Verification items for the finished model (mm, model axes). Round coordinates to 2 decimals unless told otherwise and drop trailing zeros. Loops run counter-clockwise (first coordinate to the right, second up) from the corner with the lowest first, then second, coordinate; pieces in that order, holes last. Notation, with made-up numbers: M -15,86 L 3,86 A18 cw 3,98 Z; hole C -39,35.25 d10. An arc over 180 degrees is marked long. Answer as CSV lines item,"result".
```python
from build123d import *
from OCP.BRepFilletAPI import BRepFilletAPI_MakeChamfer

# Parameters (mm, degrees)
BOSS_EXTRUDE1_DEPTH = 2.4
SKETCH2_R           = 2
CUT_EXTRUDE1_DEPTH  = 31.907209919
CHAMFER1_SIZE       = 2.38
CHAMFER1_SIZE2      = 1.109812226
SKETCH3_R           = 12.7
SKETCH3_R_2         = 11.375
BOSS_EXTRUDE2_DEPTH = 18
CUT_EXTRUDE2_START  = -30
SKETCH4_R           = 11.375
CUT_EXTRUDE2_DEPTH  = 30
CHAMFER2_SIZE       = 2.4293521
CHAMFER2_SIZE_2     = 3
CHAMFER3_SIZE       = 1.619568066
CHAMFER3_SIZE_2     = 2
CUT_EXTRUDE3_DEPTH  = 37.954778273


with BuildPart() as part:
    # Sketch1 → Boss-Extrude1 (new body)
    with BuildSketch(Plane.XY):
        with BuildLine():
            Line((6.35, 28.075), (-6.35, 28.075))
            ThreePointArc((-6.35, 28.075), (-10.840128061, 26.215128061), (-12.7, 21.725))
            Line((-12.7, 21.725), (-12.7, -21.725))
            ThreePointArc((-12.7, -21.725), (-10.840128061, -26.215128061), (-6.35, -28.075))
            Line((-6.35, -28.075), (6.35, -28.075))
            ThreePointArc((6.35, -28.075), (10.840128061, -26.215128061), (12.7, -21.725))
            Line((12.7, -21.725), (12.7, 21.725))
            ThreePointArc((12.7, 21.725), (10.840128061, 26.215128061), (6.35, 28.075))
        make_face()
    extrude(amount=BOSS_EXTRUDE1_DEPTH)

    # Sketch2 → Cut-Extrude1 (cut, through all)
    with BuildSketch(Plane(origin=(0, 0, 0), x_dir=(-1, 0, 0), z_dir=(0, 0, -1))):
        with Locations((-7.7, 20.1248)):
            Circle(SKETCH2_R)
        with Locations((-7.7, -20.125)):
            Circle(SKETCH2_R)
        with Locations((7.7, 20.125)):
            Circle(SKETCH2_R)
        with Locations((7.7, -20.125)):
            Circle(SKETCH2_R)
    extrude(amount=-CUT_EXTRUDE1_DEPTH, mode=Mode.SUBTRACT)

    # Chamfer1: one chamfer whose edges measure the first distance from different faces: ONE call of the kernel's chamfer builder (chamfer() names one face for all edges)
    chamfer1_edges_1 = [part.edges().sort_by_distance(p)[0] for p in [
        (-10.840128061, 26.215128061, 2.4),
    ]]
    chamfer1_side_1 = [part.faces().sort_by_distance(p)[0] for p in [
        (-10.840128061, 26.215128061, 1.2),
    ]]
    chamfer1_edges_2 = [part.edges().sort_by_distance(p)[0] for p in [
        (-12.7, 0, 2.4),
    ]]
    chamfer1_side_2 = [part.faces().sort_by_distance(p)[0] for p in [
        (-12.7, 0, 1.2),
    ]]
    chamfer1_edges_3 = [part.edges().sort_by_distance(p)[0] for p in [
        (-10.840128061, -26.215128061, 2.4),
    ]]
    chamfer1_side_3 = [part.faces().sort_by_distance(p)[0] for p in [
        (-10.840128061, -26.215128061, 1.2),
    ]]
    chamfer1_edges_4 = [part.edges().sort_by_distance(p)[0] for p in [
        (0, -28.075, 2.4),
    ]]
    chamfer1_side_4 = [part.faces().sort_by_distance(p)[0] for p in [
        (0, -28.075, 1.2),
    ]]
    chamfer1_edges_5 = [part.edges().sort_by_distance(p)[0] for p in [
        (10.840128061, -26.215128061, 2.4),
    ]]
    chamfer1_side_5 = [part.faces().sort_by_distance(p)[0] for p in [
        (10.840128061, -26.215128061, 1.2),
    ]]
    chamfer1_edges_6 = [part.edges().sort_by_distance(p)[0] for p in [
        (12.7, 0, 2.4),
    ]]
    chamfer1_side_6 = [part.faces().sort_by_distance(p)[0] for p in [
        (12.7, 0, 1.2),
    ]]
    chamfer1_edges_7 = [part.edges().sort_by_distance(p)[0] for p in [
        (10.840128061, 26.215128061, 2.4),
    ]]
    chamfer1_side_7 = [part.faces().sort_by_distance(p)[0] for p in [
        (10.840128061, 26.215128061, 1.2),
    ]]
    chamfer1_edges_8 = [part.edges().sort_by_distance(p)[0] for p in [
        (0, 28.075, 2.4),
    ]]
    chamfer1_side_8 = [part.faces().sort_by_distance(p)[0] for p in [
        (0, 28.075, 1.2),
    ]]
    chamfer1 = BRepFilletAPI_MakeChamfer(part.part.solid().wrapped)
    for e in chamfer1_edges_1:
        chamfer1.Add(CHAMFER1_SIZE, CHAMFER1_SIZE2, e.wrapped, chamfer1_side_1[0].wrapped)  # the first distance lies on this face
    for e in chamfer1_edges_2:
        chamfer1.Add(CHAMFER1_SIZE, CHAMFER1_SIZE2, e.wrapped, chamfer1_side_2[0].wrapped)  # the first distance lies on this face
    for e in chamfer1_edges_3:
        chamfer1.Add(CHAMFER1_SIZE, CHAMFER1_SIZE2, e.wrapped, chamfer1_side_3[0].wrapped)  # the first distance lies on this face
    for e in chamfer1_edges_4:
        chamfer1.Add(CHAMFER1_SIZE, CHAMFER1_SIZE2, e.wrapped, chamfer1_side_4[0].wrapped)  # the first distance lies on this face
    for e in chamfer1_edges_5:
        chamfer1.Add(CHAMFER1_SIZE, CHAMFER1_SIZE2, e.wrapped, chamfer1_side_5[0].wrapped)  # the first distance lies on this face
    for e in chamfer1_edges_6:
        chamfer1.Add(CHAMFER1_SIZE, CHAMFER1_SIZE2, e.wrapped, chamfer1_side_6[0].wrapped)  # the first distance lies on this face
    for e in chamfer1_edges_7:
        chamfer1.Add(CHAMFER1_SIZE, CHAMFER1_SIZE2, e.wrapped, chamfer1_side_7[0].wrapped)  # the first distance lies on this face
    for e in chamfer1_edges_8:
        chamfer1.Add(CHAMFER1_SIZE, CHAMFER1_SIZE2, e.wrapped, chamfer1_side_8[0].wrapped)  # the first distance lies on this face
    add(Compound.cast(chamfer1.Shape()), mode=Mode.REPLACE)

    # Sketch3 → Boss-Extrude2 (add)
    with BuildSketch(Plane(origin=(0, 0, 0), x_dir=(-1, 0, 0), z_dir=(0, 0, -1))):
        Circle(SKETCH3_R)
        Circle(SKETCH3_R_2, mode=Mode.SUBTRACT)
    extrude(amount=BOSS_EXTRUDE2_DEPTH)

    # Sketch4 → Cut-Extrude2 (cut)
    with BuildSketch(Plane(origin=(0, 0, 0), x_dir=(-1, 0, 0), z_dir=(0, 0, -1)).offset(CUT_EXTRUDE2_START)):
        Circle(SKETCH4_R)
    extrude(amount=CUT_EXTRUDE2_DEPTH, mode=Mode.SUBTRACT)

    # Chamfer2
    # the kernel refuses this chamfer: 3, 2.4293521 mm, written as the material it takes off along each edge
    with BuildSketch(Plane(origin=(7.7, -20.125, 2.4), x_dir=(-1, 0, 0), z_dir=(0, -1, 0))) as chamfer2_piece_1:
        Polygon((2 + CHAMFER2_SIZE, 0), (2, CHAMFER2_SIZE_2), (2, 0), align=None)
    revolve(axis=Axis((7.7, -20.125, 2.4), (0, 0, -1)), mode=Mode.SUBTRACT)
    with BuildSketch(Plane(origin=(-7.7, -20.125, 2.4), x_dir=(-1, 0, 0), z_dir=(0, -1, 0))) as chamfer2_piece_2:
        Polygon((2 + CHAMFER2_SIZE, 0), (2, CHAMFER2_SIZE_2), (2, 0), align=None)
    revolve(axis=Axis((-7.7, -20.125, 2.4), (0, 0, -1)), mode=Mode.SUBTRACT)
    with BuildSketch(Plane(origin=(7.7, 20.1248, 2.4), x_dir=(-1, 0, 0), z_dir=(0, -1, 0))) as chamfer2_piece_3:
        Polygon((2 + CHAMFER2_SIZE, 0), (2, CHAMFER2_SIZE_2), (2, 0), align=None)
    revolve(axis=Axis((7.7, 20.1248, 2.4), (0, 0, -1)), mode=Mode.SUBTRACT)
    with BuildSketch(Plane(origin=(-7.7, 20.125, 2.4), x_dir=(-1, 0, 0), z_dir=(0, -1, 0))) as chamfer2_piece_4:
        Polygon((2 + CHAMFER2_SIZE, 0), (2, CHAMFER2_SIZE_2), (2, 0), align=None)
    revolve(axis=Axis((-7.7, 20.125, 2.4), (0, 0, -1)), mode=Mode.SUBTRACT)

    # Chamfer3
    # the kernel refuses this chamfer: 2, 1.619568066 mm, written as the material it takes off along each edge
    with BuildSketch(Plane(origin=(0, 0, 2.4), x_dir=(-1, 0, 0), z_dir=(0, 1, 0))) as chamfer3_piece_1:
        Polygon((11.375 + CHAMFER3_SIZE, 0), (11.375, -CHAMFER3_SIZE_2), (11.375, 0), align=None)
    revolve(axis=Axis((0, 0, 2.4), (0, 0, 1)), mode=Mode.SUBTRACT)

    # Sketch5 → Cut-Extrude3 (cut, through all)
    with BuildSketch(Plane(origin=(0, 0, -18), x_dir=(-1, 0, 0), z_dir=(0, 0, -1))):
        with BuildLine():
            Line((-0.85, 11.343197301), (-0.85, 12.75))
            Line((-0.85, 12.75), (0.85, 12.75))
            Line((0.85, 12.75), (0.85, 11.343197301))
            ThreePointArc((0.85, 11.343197301), (0, 11.375), (-0.85, 11.343197301))
        make_face()
    extrude(amount=-CUT_EXTRUDE3_DEPTH, mode=Mode.SUBTRACT)


solid = part.part
```
1) Section check A-A (x = 0). Record the cut outline in (y, z) (3 decimals), plus the area to 3 significant figures.
Here are the results:
outline,"M -28.075,0 L -12.7,0 L -12.7,-18 L -11.375,-18 L -11.375,0.4 L -12.995,2.4 L -26.965,2.4 L -28.075,0.02 Z; M 12.75,0 L 28.075,0 L 28.075,0.02 L 26.965,2.4 L 12.995,2.4 L 12.75,2.098 Z"
area,"96.4 mm^2"
2) Draft check along Y on faces 1 (the conical face through (-4.91, 20.25, 0.38)), 2 (the flat face through (0, 19, 2.4)), 3 (the flat face through (0.09, 27.51, 1.23)). Enter one of: +Y half, -Y half, draft (parallel to the pull), parting line (faces both ways), or undercut.
Here are the results:
face 1,"undercut"
face 2,"draft"
face 3,"+Y half"
3) Material ranges on probe 1 along X at (y, z) = (20, 0.5); probe 2 along X at (y, z) = (0, -5.75) (3 decimals); probe 3 along X at (y, z) = (-4.5, -12), recorded low to high.
Here are the results:
probe 1,"x = -12.48 to -10.59, -4.81 to 4.81, 10.59 to 12.48"
probe 2,"x = -12.7 to -11.375, 11.375 to 12.7"
probe 3,"x = -11.88 to -10.45, 10.45 to 11.88"
4) Go/stop test with flat-tipped pins: pin 1 (10 mm diameter, centred on x = 7.5, y = -20.5, fed in from -Z); pin 2 (1.5 mm diameter, centred on y = 12, z = -5, fed in from -X); pin 3 (3 mm diameter, centred on x = -8, z = -2, fed in from +Y). Record where each tip stops, or that it passes through.
Here are the results:
pin 1,"stops at z = 0"
pin 2,"stops at x = -5.89"
pin 3,"stops at y = 10.91"
5) Section check C-C (x = -7.7). State how many separate pieces and enclosed holes the cut face has, plus the area to 3 significant figures.
Here are the results:
separate pieces,"4"
enclosed holes,"0"
area,"116 mm^2"
6) Section check B-B (z = -8). Record the cut outline in (x, y) (3 decimals).
Here are the results:
outline,"M -0.85,11.343 L -0.85,12.672 A12.7 ccw long 0.85,12.672 L 0.85,11.343 A11.375 cw long Z"
